```python
from build123d import *

# Parameters (mm, degrees)
BOSS_EXTRUDE4_DEPTH = 16
CUT_EXTRUDE1_DEPTH  = 16
SKETCH4_R           = 1.5
CUT_EXTRUDE3_DEPTH  = 16
SKETCH6_R           = 4
CUT_EXTRUDE4_DEPTH  = 134.582030626


with BuildPart() as part:
    # Sketch1 → Boss-Extrude4 (new body)
    with BuildSketch(Plane(origin=(0, 0, 0), x_dir=(1, 0, 0), z_dir=(0, 1, 0))):
        with BuildLine():
            Line((-101.232266869, 84.812685314), (-41.738030485, 6.78745727))
            ThreePointArc((-41.738030485, 6.78745727), (-40.683381354, 5.917890449), (-39.352420031, 5.606485241))
            Line((-39.352420031, 5.606485241), (23.167405683, 5.606485241))
            ThreePointArc((23.167405683, 5.606485241), (23.874512464, 5.313592022), (24.167405683, 4.606485241))
            Line((24.167405683, 4.606485241), (24.167405683, 2.606485241))
            ThreePointArc((24.167405683, 2.606485241), (23.874512464, 1.89937846), (23.167405683, 1.606485241))
            Line((23.167405683, 1.606485241), (-102.832594317, 1.606485241))
            ThreePointArc((-102.832594317, 1.606485241), (-104.95391466, 2.485164898), (-105.832594317, 4.606485241))
            Line((-105.832594317, 4.606485241), (-105.832594317, 5.6))
            Line((-105.832594317, 5.6), (-105.832594317, 84.6))
            ThreePointArc((-105.832594317, 84.6), (-105.539701098, 85.307106781), (-104.832594317, 85.6))
            Line((-104.832594317, 85.6), (-102.822673838, 85.6))
            ThreePointArc((-102.822673838, 85.6), (-101.93536629, 85.392396528), (-101.232266869, 84.812685314))
        make_face()
    extrude(amount=BOSS_EXTRUDE4_DEPTH)

    # Sketch2 → Cut-Extrude1 (cut)
    with BuildSketch(Plane(origin=(0, 16, 0), x_dir=(1, 0, 0), z_dir=(0, 1, 0))):
        Polygon((-101.761672648, 5.67740691), (-46.376523222, 5.67740691), (-101.761672648, 79.266350208), align=None)
    extrude(amount=-CUT_EXTRUDE1_DEPTH, mode=Mode.SUBTRACT)

    # Sketch4 → Cut-Extrude3 (cut)
    with BuildSketch(Plane.XY.offset(-1.606485241)):
        with Locations((9.667405683, 8)):
            Circle(SKETCH4_R)
        with Locations((-56.332594317, 8)):
            Circle(SKETCH4_R)
    extrude(amount=-CUT_EXTRUDE3_DEPTH, mode=Mode.SUBTRACT)

    # Sketch6 → Cut-Extrude4 (cut, through all)
    with BuildSketch(Plane(origin=(0, 0, -5.67740691), x_dir=(-1, 0, 0), z_dir=(0, 0, -1))):
        with Locations(Location((56.297582792, 8, 0), (0, 0, 180))):
            Circle(SKETCH6_R)
    extrude(amount=CUT_EXTRUDE4_DEPTH, mode=Mode.SUBTRACT)


solid = part.part
```
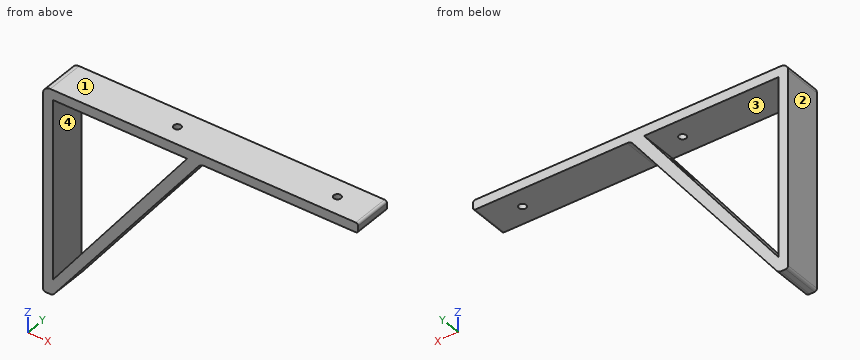
Build history of the part. All positions in model axes, mm. Face numbers are marked on the shaded views. Round coordinates to 2 decimals unless told otherwise and drop trailing zeros. Loops run counter-clockwise (first coordinate to the right, second up) from the corner with the lowest first, then second, coordinate; pieces in that order, holes last.
Item 1: Saw through at A-A (y = 14.25). List the corners of the cut face in (x, z).
Item 2: Saw through at B-B (z = -51). List the corners of the cut face in (x, y).
Item 3: Saw through at C-C (y = 8). List the corners of the cut face in (x, z).
Item 4: Pin check, flat tips, straight feed: P1, Ø5, axis at y = 9.5, z = -53, coming from the +X side; P2, Ø1, axis at x = -77.5, y = 13, coming from the -Z side; P3, Ø5, axis at x = -56.3, y = 8, coming from the +Z side; P4, Ø4, axis at x = 9.67, y = 8, coming from the -Z side. Stop position of each tip, or through.
Item 5: Saw through at D-D (x = -75). List the corners of the cut face in (y, z).
Item 6: Drill centre lines: line 1 along Z through (x, y) = (-27, 13); line 2 along Z through (x, y) = (-86, 12); line 3 along X through (y, z) = (14.25, -45). Where is each one in solid material? Low to high.
Item 7: Two-plate mould, pull along X, no slides. Class the marked faces 1, 2, 3 and 4: released by +X, released by -X, zero draft, split by the parting line, or undercut.
Worked answers:
1. outline: (-105.83, -84.6) arc R1 ccw to (-104.83, -85.6) - (-102.82, -85.6) arc R2 ccw to (-101.23, -84.81) - (-41.74, -6.79) arc R3 cw to (-39.35, -5.61) - (23.17, -5.61) arc R1 ccw to (24.17, -4.61) - (24.17, -2.61) arc R1 ccw to (23.17, -1.61) - (-102.83, -1.61) arc R3 ccw to (-105.83, -4.61) - close; hole (-101.76, -79.27) - (-46.38, -5.68) - (-101.76, -5.68) - close
2. outline: (-105.83, 0) - (-101.76, 0) - (-101.76, 16) - (-105.83, 16) - close; (-80.49, 0) - (-75.45, 0) - (-75.45, 16) - (-80.49, 16) - close
3. outline: (-105.83, -84.6) arc R1 ccw to (-104.83, -85.6) - (-102.82, -85.6) arc R2 ccw to (-101.23, -84.81) - (-60.3, -31.13) - (-60.3, -24.17) - (-101.76, -79.27) - (-101.76, -5.68) - (-57.83, -5.68) - (-57.83, -1.61) - (-102.83, -1.61) arc R3 ccw to (-105.83, -4.61) - close; (-54.83, -5.68) - (-46.38, -5.68) - (-52.3, -13.54) - (-52.3, -20.64) - (-41.74, -6.79) arc R3 cw to (-39.35, -5.61) - (8.17, -5.61) - (8.17, -1.61) - (-54.83, -1.61) - close; (11.17, -5.61) - (23.17, -5.61) arc R1 ccw to (24.17, -4.61) - (24.17, -2.61) arc R1 ccw to (23.17, -1.61) - (11.17, -1.61) - close
4. P1: stops at x = -75.07
4. P2: stops at z = -54.34
4. P3: stops at z = -1.61
4. P4: stops at z = -5.61
5. outline: (0, -50.41) - (16, -50.41) - (16, -43.71) - (0, -43.71) - close; (0, -5.68) - (16, -5.68) - (16, -1.61) - (0, -1.61) - close
6. line 1: z = -5.61 to -1.61
6. line 2: z = -64.84 to -58.32, -5.68 to -1.61
6. line 3: x = -105.83 to -101.76, -75.97 to -70.88
7. face 1: zero draft
7. face 2: released by -X
7. face 3: undercut
7. face 4: undercut
